Read the model definition and answer for the solid it produces. Units are mm, in the model's axes. A direction names the side the tool comes from. Round coordinates to 2 decimals unless told otherwise and drop trailing zeros. Write each loop counter-clockwise with the first axis right and the second up, starting at its lowest first coordinate (ties: lowest second). Pieces come first, ordered by that corner, then holes. Notation, with made-up numbers: M 89.25,-18 L 120.25,-18 A22 ccw 120.25,20 Z; hole C 13,36.5 d8. An arc over 180 degrees is marked long. Use one line per item in the form item = value. Start each with the question number.
Autodesk Inventor part; units mm, degrees
ref_plane "Arbeitsebene2" through (0, 10, 0) normal (0, 1, 0) x (-1, 0, 0)
ref_plane "YZ Plane" through (0, 0, 0) normal (1, 0, 0) x (0, 1, 0)
ref_plane "XY Plane" through (0, 0, 0) normal (0, 0, 1) x (1, 0, 0)
sketch "Skizze1" plane through (0, 0, 0) normal (0, 0, 1) x (1, 0, 0)
  line L0 (20, 16.3) -> (20, 0)
  line L1 (20, 0) -> (-20, 0)
  line L2 (-20, 0) -> (-20, 16.3)
  line L3 (-16, 8.4971) -> (-16, 1.5701)
  line L4 (-16, 1.5701) -> (16, 1.5701)
  line L5 (16, 1.5701) -> (16, 8.4971)
  line L6 (-20, 16.3) -> (-17.85, 16.3)
  line L7 (20, 16.3) -> (17.85, 16.3)
  arc A0 (-16, 8.4971) -> (16, 8.4971) centre (0, 30.4255) ccw
  arc A1 (-17.85, 16.3) -> (17.85, 16.3) centre (0, 25.395) ccw
  line L8 (2.1309, 0) -> (0, 0)
  line L9 (0, 16.2928) -> (2.1309, 16.2928)
  line L10 (2.1309, 16.2928) -> (2.1309, 0)
  line L11 (2.1309, 0) -> (0, 0)
  line L12 (0, 0) -> (0, 16.2928)
  line L13 (37.8691, 16.2928) -> (40, 16.2928)
  line L14 (40, 16.2928) -> (40, 0)
  line L15 (40, 0) -> (37.8691, 0)
  line L16 (37.8691, 0) -> (37.8691, 16.2928)
  line L17 (0, 0) -> (40, 0)
  line L18 (0, 0) -> (0, 12.8953)
  line L19 (40, 0) -> (40, 79)
  arc A2 (2.1309, 16.2928) -> (37.8691, 16.2928) centre (20, 25.8644) ccw
  line L20 (6.1071, 11.1028) -> (5.3563, 11.7632)
  point P0 (0, 8.1464)
  dimension "d27" = 40
  dimension "d28" = 4
  dimension "d58" = 16.3
  dimension "d60" = 126
  dimension "d61" = 2.15
  dimension "d62" = 2.1309
extrude "Extrusion1" add sketch "Skizze1" along normal blind 25 contours L0 A2 L5 A0 A1 L7 | L0 L1 L10 L4 L5 A2 | A2 A0 L10 A1 | L1 L12 L4 L10 | L10 A0 L12 A1 | L1 L2 L6 A1 L12 A0 L3 L4
sketch "Skizze2" plane through (-20, 16.3, 0) normal (0, 1, 0) x (1, 0, 0)
  line L0 (2.15, 0) -> (0, 0)
  line L1 (0, 0) -> (0, -25)
  line L2 (2.15, -25) -> (0, -25)
  line L3 (2.15, 0) -> (2.15, -25)
  point P0 (20, 0)
extrude "Extrusion2" add sketch "Skizze2" along normal blind 3
sketch "Skizze3" plane through (17.85, 16.3, 0) normal (0, 1, 0) x (1, 0, 0)
  line L0 (2.15, 0) -> (0, 0)
  line L1 (0, 0) -> (0, -25)
  line L2 (2.15, -25) -> (0, -25)
  line L3 (2.15, 0) -> (2.15, -25)
  point P0 (-17.85, 0)
ref_plane "Arbeitsebene2" through (0, 10, 0) normal (0, 1, 0) x (-1, 0, 0)
extrude "Extrusion3" add sketch "Skizze3" along normal blind 3
sketch "Skizze4" plane through (0, 10, 0) normal (0, 1, 0) x (-1, 0, 0)
  line L0 (-17.85, 0) -> (-17.85, 25)
  line L1 (-17.85, 0) -> (17.85, 0)
  line L2 (17.85, 0) -> (17.85, 25)
  line L3 (-17.85, 25) -> (17.85, 25)
  line L4 (-17.85, 0) -> (-17.85, 25)
  line L5 (-17.85, 11.4) -> (17.85, 11.4)
  line L6 (-17.85, 13.65) -> (17.85, 13.65)
  line L7 (-17.85, 16.4) -> (17.85, 16.4)
  line L8 (-17.85, 18.65) -> (17.85, 18.65)
  line L9 (-17.85, 25) -> (-20, 25)
  point P0 (0, 0)
  point P1 (-17.85, 13.65)
  point P2 (-17.85, 11.4)
  point P3 (-17.85, 18.65)
  point P4 (-17.85, 16.4)
  dimension "d13" = 2.25
  dimension "d14" = 2.25
  dimension "d15" = 25
  dimension "d16" = 2.75
  dimension "d36" = 6.35
extrude "Extrusion4" cut sketch "Skizze4" along normal mid plane 14 contours L0 L6 L2 L5 | L0 L8 L2 L7
fillet "Rundung2" radius 2 2 edges at (-20, 19.3, 12.5) (20, 19.3, 12.5)
sketch "Skizze5" plane through (-16, 1.5701, 0) normal (1, 0, 0) x (0, 0, -1)
  line L0 (0, 0) -> (0, 6.927)
  line L1 (0, 6.927) -> (-25, 6.927)
  line L2 (-25, 0) -> (-25, 6.927)
  line L3 (0, 0) -> (-25, 0)
  point P0 (0, -1.5701)
sketch "Skizze12" plane through (-20, 0, 0) normal (-1, 0, 0) x (0, 0, 1)
  line L0 (0, 0) -> (25, 0)
  line L1 (18.65, 6.5) -> (18.65, 12)
  line L2 (13.65, 6.5) -> (13.65, 12)
  line L3 (18.65, 12) -> (16.4, 12)
  line L4 (16.4, 12) -> (16.4, 0)
  line L5 (16.4, 0) -> (18.65, 0)
  line L6 (18.65, 0) -> (18.65, 12)
  line L7 (13.65, 12) -> (11.4, 12)
  line L8 (11.4, 12) -> (11.4, 0)
  line L9 (11.4, 0) -> (13.65, 0)
  line L10 (13.65, 0) -> (13.65, 12)
  point P0 (27, 0)
  point P1 (13.65, 0)
  point P2 (18.65, 0)
  dimension "d52" = 2.75
  dimension "d54" = 2.25
  dimension "d55" = 2.25
extrude "Extrusion10" cut sketch "Skizze12" against normal blind 5
sketch "Skizze13" plane through (0, 0, 25) normal (0, 0, 1) x (1, 0, 0)
  arc A0 (20, 17.3) -> (17.85, 19.3) centre (18, 17.3) ccw
  line L0 (17.85, 16.3) -> (17.85, 19.3)
  arc A1 (-17.85, 16.3) -> (17.85, 16.3) centre (0, 25.395) ccw
  line L1 (-17.85, 16.3) -> (-17.85, 19.3)
  arc A2 (-17.85, 19.3) -> (-20, 17.3) centre (-18, 17.3) ccw
  line L2 (-20, 0) -> (-20, 17.3)
  line L3 (-20, 0) -> (20, 0)
  line L4 (20, 0) -> (20, 17.3)
  arc A3 (-16, 8.4971) -> (16, 8.4971) centre (0, 30.4255) ccw
  line L5 (16, 8.4971) -> (16, 1.5701)
  line L6 (16, 1.5701) -> (-16, 1.5701)
  line L7 (-16, 1.5701) -> (-16, 8.4971)
  point P0 (0, 0)
properties part number "Gehäuse_Kurve" material "ABS-Kunststoff"
Q1. Straight lines are drawn through the part: line 1 (Z direction, x = -6.5, y = 4.5); line 2 (X direction, y = 16.75, z = 8); line 3 (X direction, y = 7, z = 3.5). For each, find the intervals that lie inside material, in ascending order. Write a range as [from, to].
Q2. Each of these flat-tipped pins is pushed along its axis until it touches: pin 1 Ø0.5 at (y, z) = (1, 13) entering from -X; pin 2 Ø7.5 at (x, z) = (-0.5, 8.5) entering from +Y; pin 3 Ø8 at (x, z) = (6.5, 17.5) entering from +Y. Where does it stop, or does it pass through?
Q3. Find section A-A on x = 0. Write down the section's boundary in (y, z).
Q4. For a pull along X with two mould halves and no side action, classify faces 4 (the face through (-15, 1, 18)), 5 (the face through (17, 3, 13)), 6 (the face through (-17.85, 17, 12)) as +X half, -X half, draft (parallel to the pull), parting line (faces both ways), or undercut.
Q5. Find section D-D on z = 12.5. Write down the section's boundary in (x, y).
Q6. A tool of negligible diameter and unlimited length cuts with its end or side. For faces 1 (the face through (0, 1.57, 12)), 2 (the face through (-20, 9, 10)), 3 (the face through (17.85, 15, 12)), from which of +Z, -Z, +X, -X, +Y, -Y can it reach the whole face along a straight path? Write none if from no direction.
Q7. Find section C-C on y = 15.5. Write down the section's boundary in (x, z), and give its area (3 significant figures).
Response:
q1.line_1 = [0, 11.4], [13.65, 16.4], [18.65, 25]
q1.line_2 = [-20, -17.85], [17.85, 20]
q1.line_3 = [-20, -16], [-13.71, -7.94], [7.94, 13.71], [16, 20]
q2.pin_1 = -15
q2.pin_2 = 5.82
q2.pin_3 = 8.24
q3.outline = M 0,0 L 1.57,0 L 1.57,25 L 0,25 Z; M 3.28,0 L 5.36,0 L 5.36,11.4 L 3.28,11.4 Z; M 3.28,13.65 L 5.36,13.65 L 5.36,16.4 L 3.28,16.4 Z; M 3.28,18.65 L 5.36,18.65 L 5.36,25 L 3.28,25 Z
q4.face_4 = -X half
q4.face_5 = draft
q4.face_6 = undercut
q5.outline = M -20,12 L -17.85,12 L -17.85,19.3 L -18,19.3 A2 ccw -20,17.3 Z; M -15,0 L 20,0 L 20,17.3 A2 ccw 18,19.3 L 17.85,19.3 L 17.85,3 L 16,3 L 16,1.57 L -15,1.57 Z
q6.face_1 = +Z, -Z
q6.face_2 = +Z, -Z, -X, +Y, -Y
q6.face_3 = +Y
q7.outline = M -20,0 L -17.42,0 L -17.42,11.4 L -17.85,11.4 L -17.85,13.65 L -17.42,13.65 L -17.42,16.4 L -17.85,16.4 L -17.85,18.65 L -17.42,18.65 L -17.42,25 L -20,25 Z; M 17.42,0 L 20,0 L 20,25 L 17.42,25 L 17.42,18.65 L 17.85,18.65 L 17.85,16.4 L 17.42,16.4 L 17.42,13.65 L 17.85,13.65 L 17.85,11.4 L 17.42,11.4 Z
q7.area = 125 mm²
